from build123d import *

# Parameters (mm, degrees)
F1_DEPTH = 19.05
F3_R     = 1.27


# Not quite as in the source:
# - a feature of the source that left no trace in its solid (it failed there, or was rolled back) is left out


with BuildPart() as f1:
    # F0 (on Top) → F1 (new body, symmetric)
    with BuildSketch(Plane.XY):
        with BuildLine():
            Line((-38.3560955603, 23.021564283), (0, -55.7964481413))
            Line((0, -55.7964481413), (38.3560955603, 23.021564283))
            ThreePointArc((38.3560955603, 23.021564283), (0, 31.8589518587), (-38.3560955603, 23.021564283))
        make_face()
    extrude(amount=F1_DEPTH, both=True)

    # F3
    f3_edges = [f1.edges().sort_by_distance(p)[0] for p in [
        (0, -55.796448, 0),
        (38.356096, 23.021564, 0),
        (-38.356096, 23.021564, 0),
        (-19.178048, -16.387442, -19.05),
        (-19.178048, -16.387442, 19.05),
        (0, 31.858952, -19.05),
        (0, 31.858952, 19.05),
        (19.178048, -16.387442, 19.05),
        (19.178048, -16.387442, -19.05),
    ]]
    fillet(f3_edges, radius=F3_R)


solid = f1.part
Source: CAD feature listing. Evaluate the final solid. Frame: model axes, mm. Give positions to 0.01 mm unless a question says otherwise; leave off trailing zeros. Write each loop counter-clockwise with the first axis right and the second up, starting at its lowest first coordinate (ties: lowest second). Pieces come first, ordered by that corner, then holes. Notation, with made-up numbers: M 74,55.25 L 129,55.25 A23 cw 129,92.25 Z; hole C -22.75,-9 d2. An arc over 180 degrees is marked long. Answer as a JSON object with one key per item and string values.
Q1. Cut plane A-A, the plane z = -1. Return the cut outline in (x, y), then the cut area to 3 significant figures.
Geometry check:
{"outline": "M -37.8,21.87 L -1.14,-53.45 A1.27 ccw 1.14,-53.45 L 37.8,21.87 A1.27 ccw 37.19,23.58 A87.66 ccw -37.19,23.58 A1.27 ccw Z", "area": "3,480 mm^2"}
Q2. Ray query, line 1 along Y through (x, z) = (9.5, 7); line 2 along X through (y, z) = (-30.5, 7); line 3 along Y through (x, z) = (-5.5, 16). Return the intervals inside material, ascending.
Geometry check:
{"line 1": "y = -36.27 to 31.34", "line 2": "x = -12.31 to 12.31", "line 3": "y = -44.49 to 31.69"}
Q3. Contact query for flat-ended pins moving along their axis: P1, Ø1.5, axis at y = -3.5, z = -9, coming from the +X side; P2, Ø1, axis at y = -26.5, z = -15, coming from the +X side; P3, Ø5, axis at y = 15.5, z = 7.5, coming from the +X side. Output: stop coordinate, or through.
Geometry check:
{"P1": "stops at x = 25.81", "P2": "stops at x = 14.5", "P3": "stops at x = 35.91"}
